Model file for the job. Use its own axes, mm. A direction names the side the tool comes from. Coordinates: 2 decimals unless noted, no trailing zeros. Write each loop counter-clockwise with the first axis right and the second up, starting at its lowest first coordinate (ties: lowest second). Pieces come first, ordered by that corner, then holes. Notation, with made-up numbers: M -10.5,30.5 L -0.5,30.5 A16 ccw -0.5,36.5 Z; hole C 71,53.25 d5. An arc over 180 degrees is marked long. Answer in a Markdown table with one row per item. Add a question column.
Autodesk Inventor part; units mm, degrees
ref_plane "YZ Plane" through (0, 0, 0) normal (1, 0, 0) x (0, 1, 0)
ref_plane "XZ Plane" through (0, 0, 0) normal (0, 1, 0) x (-1, 0, 0)
ref_plane "XY Plane" through (0, 0, 0) normal (0, 0, 1) x (1, 0, 0)
sketch "Sketch1" plane through (0, 0, 0) normal (1, 0, 0) x (0, 1, 0)
  line L0 (0, 0) -> (0, 2)
  line L1 (0, 1) -> (9, 1) construction
  line L2 (10, 2) -> (9, 1)
  line L3 (9, 1) -> (10, 0)
  line L4 (10, 2) -> (0, 2)
  line L5 (10, 0) -> (0, 0)
  dimension "d0" = 2
  dimension "d2" = 1
  dimension "d3" = 1
  dimension "d4" = 1
  dimension "d5" = 10
revolve "Revolution1" add sketch "Sketch1" angle 360 about axis through (0, 0, 0) along (0, 0, 1)
fillet "Fillet1" radius 0.1 2 edges at (0, -10, 2) (0, -10, 0)
sketch "Sketch2" plane through (0, 0, 2) normal (0, 0, 1) x (1, 0, 0)
  circle A0 centre (0, 0) radius 9 construction
  line L0 (-1.6, 1.6) -> (1.6, 1.6)
  line L1 (1.6, 1.6) -> (1.6, -1.6)
  line L2 (1.6, -1.6) -> (-1.6, -1.6)
  line L3 (-1.6, -1.6) -> (-1.6, 1.6)
  line L4 (-1.6, 1.6) -> (1.6, -1.6) construction
  line L5 (1.6, 1.6) -> (-1.6, -1.6) construction
  dimension "d8" = 3.2
  dimension "d9" = 3.2
extrude "Extrusion1" cut sketch "Sketch2" against normal through all
equation "\"d3\" = d2"
equation "\"d4\" = d3"
equation "\"d9\" = d8"
properties part number "pulley" material "PC/ABS Plastic"
1) Drill centre lines: probe 1 along Y at (x, z) = (-1, 1.3); probe 2 along Y at (x, z) = (-0.5, 1.3); probe 3 along Y at (x, z) = (-2.5, 0.85). Where is each one in solid material? Low to high.
2) Slice it at C-C (z = 0.55). Give the cut face in (x, y).
3) Two-plate mould, pull along Y, no slides. Class faces 3 (the face through (2, 0, 0)), 4 (the face through (0, 1.6, 1)): released by +Y, released by -Y, zero draft, split by the parting line, or undercut.
4) Slice it at A-A (y = 0). Give the cut face in (x, z), then the cut area to 3 significant figures.
5) Flat gauge pins, fed straight in: pin 1 Ø1 at (x, z) = (0.5, 1) entering from -Y; pin 2 Ø1 at (y, z) = (0.5, 0.5) entering from +X; pin 3 Ø1 at (y, z) = (-1.5, 1) entering from -X. Where does each tip first touch, or does it go through?
6) Which spindle directions (+Z, -Z, +X, -X, +Y, -Y) get a long thin tool onto all of the face, cutting with end or side? Do faces 1 (the face through (2, 0, 2)), 2 (the face through (1.6, 0, 1)). Say none if no direction does.
Ans:
| question | item | result |
|---|---|---|
| 1 | probe 1 | y = -9.25 to -1.6, 1.6 to 9.25 |
| 1 | probe 2 | y = -9.29 to -1.6, 1.6 to 9.29 |
| 1 | probe 3 | y = -8.8 to 8.8 |
| 2 | outline | C 0,0 d18.9; hole M -1.6,-1.6 L 1.6,-1.6 L 1.6,1.6 L -1.6,1.6 Z |
| 3 | face 3 | zero draft |
| 3 | face 4 | undercut |
| 4 | outline | M -9.83,0.17 A0.1 ccw -9.76,0 L -1.6,0 L -1.6,2 L -9.76,2 A0.1 ccw -9.83,1.83 L -9,1 Z; M 1.6,0 L 9.76,0 A0.1 ccw 9.83,0.17 L 9,1 L 9.83,1.83 A0.1 ccw 9.76,2 L 1.6,2 Z |
| 4 | area | 31.6 mm2 |
| 5 | pin 1 | stops at y = -9.49 |
| 5 | pin 2 | stops at x = 9.86 |
| 5 | pin 3 | stops at x = -9.39 |
| 6 | face 1 | +Z, +X, -X, +Y, -Y |
| 6 | face 2 | +Z, -Z |
